from build123d import *

# Parameters (mm, degrees)
SZKIC1_R                    = 3.05
DODANIE_WYCI_GNI_CIE1_DEPTH = 5
WYTNIJ_WYCI_GNI_CIE2_DEPTH  = 10
WYTNIJ_WYCI_GNI_CIE4_DEPTH  = 10
DODANIE_WYCI_GNI_CIE2_DEPTH = 5.25
OBR_T1_ANGLE                = 90
OBR_T2_ANGLE                = 90
SZKIC8_W                    = 100.07426583
SZKIC8_H                    = 50.963746487
WYTNIJ_WYCI_GNI_CIE5_DEPTH  = 23
WYTNIJ_WYCI_GNI_CIE6_DEPTH  = 2
WYTNIJ_WYCI_GNI_CIE7_DEPTH  = 2
WYTNIJ_WYCI_GNI_CIE9_DEPTH  = 5.25
ZAOKR_GLENIE2_R             = 1


# Read off the part's stored shape, not the designer's step: Obrót1, Obrót2
with BuildPart() as part:
    # Szkic1 → Dodanie-wyciągnięcie1 (new body)
    with BuildSketch(Plane.XY):
        with BuildLine():
            Line((-20, 0), (20, 0))
            Line((20, 0), (35.574751144, -15.6155831))
            ThreePointArc((35.574751144, -15.6155831), (35.476976606, -24.481579544), (26.61176868, -24.328148016))
            Line((26.61176868, -24.328148016), (12.321086207, -10))
            Line((12.321086207, -10), (-12.321086207, -10))
            Line((-12.321086207, -10), (-32.989436275, -37.090675759))
            ThreePointArc((-32.989436275, -37.090675759), (-42.12272692, -40.342590816), (-43.451924108, -30.739196396))
            Line((-43.451924108, -30.739196396), (-20, 0))
        make_face()
        with Locations((-38.879391697, -35)):
            Circle(SZKIC1_R, mode=Mode.SUBTRACT)
        with Locations((31.120608303, -20)):
            Circle(SZKIC1_R, mode=Mode.SUBTRACT)
    dodanie_wyci_gni_cie1 = extrude(amount=DODANIE_WYCI_GNI_CIE1_DEPTH)

    # Szkic3 → Wytnij-wyciągnięcie2 (cut)
    with BuildSketch(Plane(origin=(0, 0, 0), x_dir=(-1, 0, 0), z_dir=(0, 0, -1))):
        with BuildLine():
            Line((21.683047095, -8.225427037), (35.260679995, -26.209046772))
            ThreePointArc((35.260679995, -26.209046772), (34.75757763, -29.812902485), (31.153721917, -29.309800121))
            Line((31.153721917, -29.309800121), (17.576089017, -11.326180386))
            ThreePointArc((17.576089017, -11.326180386), (18.079191382, -7.722324673), (21.683047095, -8.225427037))
        make_face()
    wytnij_wyci_gni_cie2 = extrude(amount=-WYTNIJ_WYCI_GNI_CIE2_DEPTH, mode=Mode.SUBTRACT)

    # Szkic4 → Wytnij-wyciągnięcie4 (cut)
    with BuildSketch(Plane(origin=(0, 0, 0), x_dir=(-1, 0, 0), z_dir=(0, 0, -1))):
        with BuildLine():
            Line((-15.517695436, -8.06176207), (-21.039997823, -13.584064457))
            ThreePointArc((-21.039997823, -13.584064457), (-25.043667053, -13.584064457), (-25.043667053, -9.580395227))
            Line((-25.043667053, -9.580395227), (-19.521364667, -4.05809284))
            ThreePointArc((-19.521364667, -4.05809284), (-15.517695436, -4.05809284), (-15.517695436, -8.06176207))
        make_face()
    wytnij_wyci_gni_cie4 = extrude(amount=-WYTNIJ_WYCI_GNI_CIE4_DEPTH, mode=Mode.SUBTRACT)

    # Szkic5 → Dodanie-wyciągnięcie2 (add)
    with BuildSketch(Plane.XY.offset(5)):
        with BuildLine():
            Line((-1.922496946, -4.528242282), (-2.878604971, -4.259692233))
            ThreePointArc((-2.878604971, -4.259692233), (0, -2.078230062), (2.878604971, -4.259692233))
            Line((2.878604971, -4.259692233), (1.925488275, -4.527402083))
            ThreePointArc((1.925488275, -4.527402083), (0.001178609, -3.075757991), (-1.922496946, -4.528242282))
        make_face()
        with BuildLine():
            Line((-1.925488275, -5.609058042), (-2.878604971, -5.876767892))
            ThreePointArc((-2.878604971, -5.876767892), (0, -8.058230062), (2.878604971, -5.876767892))
            Line((2.878604971, -5.876767892), (1.925488275, -5.609058042))
            ThreePointArc((1.925488275, -5.609058042), (0, -7.068230062), (-1.925488275, -5.609058042))
        make_face()
    dodanie_wyci_gni_cie2 = extrude(amount=DODANIE_WYCI_GNI_CIE2_DEPTH)

    # Obrót1 outline → Obrót1 (revolve)
    with BuildSketch(Plane(origin=(0, -5.076440198, 0), x_dir=(0.7071067811865502, 0.7071067811865448, 0), z_dir=(0.7071067811865448, -0.7071067811865502, 0))):
        with BuildLine():
            ThreePointArc((2.998210136, 10.25), (3.619530479, 11.75), (2.998210136, 13.25))
            Line((2.998210136, 13.25), (2.998210136, 15.25))
            Line((2.998210136, 15.25), (1.907479051, 15.25))
            Line((1.907479051, 15.25), (1.907479051, 10.25))
            Line((1.907479051, 10.25), (2.998210136, 10.25))
        make_face()
    obr_t1 = revolve(axis=Axis((0, -5.076440198, 0), (0, 0, 1)), revolution_arc=OBR_T1_ANGLE)

    # Obrót2 outline → Obrót2 (revolve)
    with BuildSketch(Plane(origin=(0, -5.076440198, 0), x_dir=(-0.7071067811865493, -0.7071067811865457, 0), z_dir=(-0.7071067811865457, 0.7071067811865493, 0))):
        with BuildLine():
            Line((1.981789864, 15.25), (1.981789864, 10.25))
            Line((1.981789864, 10.25), (2.981789864, 10.25))
            ThreePointArc((2.981789864, 10.25), (3.603110208, 11.75), (2.981789864, 13.25))
            Line((2.981789864, 13.25), (2.981789864, 15.25))
            Line((2.981789864, 15.25), (1.981789864, 15.25))
        make_face()
    obr_t2 = revolve(axis=Axis((0, -5.076440198, 0), (0, 0, 1)), revolution_arc=OBR_T2_ANGLE)

    # Lustro4: Dodanie-wyciągnięcie1, Wytnij-wyciągnięcie2, Wytnij-wyciągnięcie4, Dodanie-wyciągnięcie2, Obrót1, Obrót2 across plane
    add(dodanie_wyci_gni_cie1.mirror(Plane(origin=(-38.879391697, -35, 0), x_dir=(1, 0, 0), z_dir=(0, 0, 1))))
    add(wytnij_wyci_gni_cie2.mirror(Plane(origin=(-38.879391697, -35, 0), x_dir=(1, 0, 0), z_dir=(0, 0, 1))), mode=Mode.SUBTRACT)
    add(wytnij_wyci_gni_cie4.mirror(Plane(origin=(-38.879391697, -35, 0), x_dir=(1, 0, 0), z_dir=(0, 0, 1))), mode=Mode.SUBTRACT)
    add(dodanie_wyci_gni_cie2.mirror(Plane(origin=(-38.879391697, -35, 0), x_dir=(1, 0, 0), z_dir=(0, 0, 1))))
    add(obr_t1.mirror(Plane(origin=(-38.879391697, -35, 0), x_dir=(1, 0, 0), z_dir=(0, 0, 1))))
    add(obr_t2.mirror(Plane(origin=(-38.879391697, -35, 0), x_dir=(1, 0, 0), z_dir=(0, 0, 1))))

    # Szkic8 → Wytnij-wyciągnięcie5 (cut)
    with BuildSketch(Plane.XY):
        with Locations((-3.506949348, -18.717463345)):
            Rectangle(SZKIC8_W, SZKIC8_H)
    extrude(amount=WYTNIJ_WYCI_GNI_CIE5_DEPTH, mode=Mode.SUBTRACT)

    # Szkic9 → Wytnij-wyciągnięcie6 (cut)
    with BuildSketch(Plane.XY.offset(-5)):
        Polygon((33.793576108, -9.633416266), (20.924371092, -22.502621281), (34.229820345, -35.808070534), (47.099025361, -22.938865519), align=None)
    extrude(amount=WYTNIJ_WYCI_GNI_CIE6_DEPTH, mode=Mode.SUBTRACT)

    # Szkic10 → Wytnij-wyciągnięcie7 (cut)
    with BuildSketch(Plane.XY.offset(-5)):
        Polygon((-30.537850877, -36.007651395), (-42.082921385, -27.199544837), (-48.802909893, -36.007651395), (-37.257839386, -44.815757953), align=None)
    extrude(amount=WYTNIJ_WYCI_GNI_CIE7_DEPTH, mode=Mode.SUBTRACT)

    # Szkic14 → Wytnij-wyciągnięcie9 (cut)
    with BuildSketch(Plane(origin=(0, 0, -10.25), x_dir=(-1, 0, 0), z_dir=(0, 0, -1))):
        with BuildLine():
            Line((-2.559394547, -2.517045651), (-1.348791372, -3.727648826))
            Line((-1.348791372, -3.727648826), (1.348791372, -3.727648826))
            Line((1.348791372, -3.727648826), (2.559394547, -2.517045651))
            ThreePointArc((2.559394547, -2.517045651), (3.408337444, -5.072577978), (2.547783661, -7.624223859))
            Line((2.547783661, -7.624223859), (1.410102537, -6.486542735))
            Line((1.410102537, -6.486542735), (-1.410102537, -6.486542735))
            Line((-1.410102537, -6.486542735), (-2.547783661, -7.624223859))
            ThreePointArc((-2.547783661, -7.624223859), (-3.611320344, -5.073039448), (-2.559394547, -2.517045651))
        make_face()
    extrude(amount=-WYTNIJ_WYCI_GNI_CIE9_DEPTH, mode=Mode.SUBTRACT)

    # Zaokrąglenie2
    zaokr_glenie2_edges = [part.edges().sort_by_distance(p)[0] for p in [
        (0, -2.078230062, -15.25),
        (0, -8.058230062, -15.25),
    ]]
    fillet(zaokr_glenie2_edges, radius=ZAOKR_GLENIE2_R - 0.0001)  # a hair under: the kernel refuses the full size


solid = part.part
Read the model definition and answer for the solid it produces. Units are mm, in the model's axes. A direction names the side the tool comes from. Round coordinates to 2 decimals unless told otherwise and drop trailing zeros. Order: outer loops, then holes, each group sorted by start corner. A loop starts at its lowest first (then second) coordinate and runs counter-clockwise, first axis right, second up.
1) Straight lines are drawn through the part: L1, parallel to X at y = -34.5, z = -1; L2, parallel to X at y = -37.5, z = -2; L3, parallel to Z at x = 25, y = -16.5. For each, find the intervals that lie inside material, in ascending order.
2) Flat-ended cylindrical pins translate along their axes: pin 1 (1.5 mm diameter, centred on y = -8.5, z = -9, fed in from +X); pin 2 (5.5 mm diameter, centred on x = -3, z = -1.5, fed in from -Y); pin 3 (1 mm diameter, centred on y = -35, z = -2, fed in from +X); pin 4 (2 mm diameter, centred on y = -29.5, z = -7.5, fed in from -X). Find the tip coordinate at first contact, or state that the pin passes through.
3) The part is cut by section A-A on x = -22.5. Write down the section's boundary in (y, z), plus the area to 3 significant figures.
4) The mould has two halves that part along Y. Classify faces 4 (the face through (-28.377, -17.091, -2.465)), 5 (the face through (15.562, -4.015, -2.465)), 6 (the face through (-0.03, -2.08, -7.59)), 7 (the face through (28, -22, -3)): released by +Y, released by -Y, zero draft, split by the parting line, or undercut.
5) The part is cut by section B-B on y = -33. Write down the section's boundary in (x, z).
6) For faces 1 (the face through (0.022, -3.076, -7.588)), 2 (the face through (-0.02, -7.06, -12.72)), 3 (the face through (27.341, -16.086, -4.014)), determine the directions among +Z, -Z, +X, -X, +Y, -Y from which every point of the face is accessible in a straight line to the end or side of a thin tool.
7) The part is cut by section C-C on x = -4. Write down the section's boundary in (y, z).
Resolved:
1. L1: x = -45.11 to -41.89, -35.87 to -31.01
1. L2: x = -44.61 to -40.63, -37.13 to -33.15
1. L3: z = -5 to 0
2. pin 1: stops at x = 1.32
2. pin 2: stops at y = -10
2. pin 3: stops at x = -31.01
2. pin 4: passes through
3. outline: (-23.34, -5) - (-17.85, -5) - (-17.85, 0) - (-23.34, 0) - close; (-9.31, -5) - (-3.28, -5) - (-3.28, 0) - (-9.31, 0) - close
3. area: 57.6 mm2
4. face 4: undercut
4. face 5: undercut
4. face 6: released by +Y
4. face 7: zero draft
5. outline: (-44.8, -3) - (-41.18, -3) - (-41.18, 0) - (-44.8, 0) - close; (-36.58, -3) - (-34.48, -3) - (-34.48, -5) - (-29.87, -5) - (-29.87, 0) - (-36.58, 0) - close
6. face 1: none
6. face 2: -Z
6. face 3: -Z, +X, -Y
7. outline: (-10, -5) - (0, -5) - (0, 0) - (-10, 0) - close
